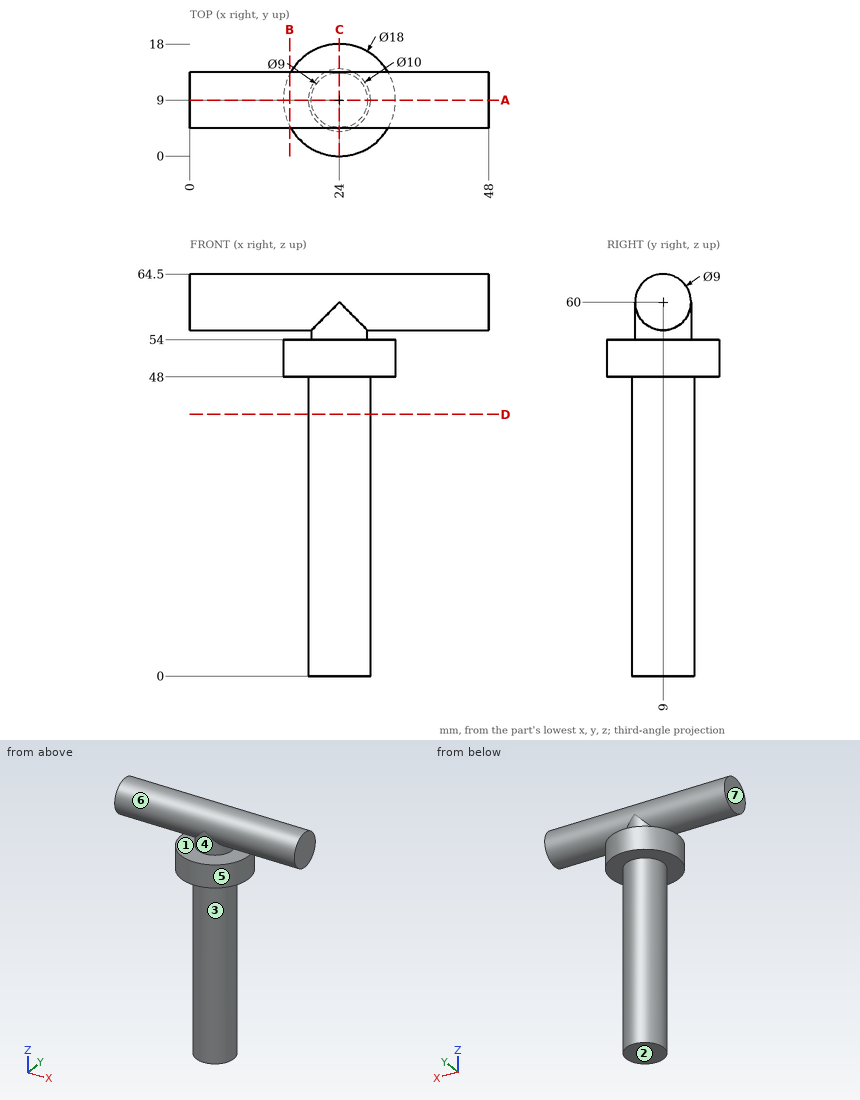
Part print with two shaded views. Sizes in mm from the minimum x, y, z corner. A direction names the side the tool comes from. Give positions to 0.01 mm unless a question says otherwise; leave off trailing zeros. Order: outer loops, then holes, each group sorted by start corner. A loop starts at its lowest first (then second) coordinate and runs counter-clockwise, first axis right, second up. Notation, with made-up numbers: M 0.5,-14.5 L 19.5,-14.5 A20 ccw 19.5,23.5 Z; hole C 16.5,38.5 d10. An arc over 180 degrees is marked long. Write item = value, one per line.
Q1. Cut at D-D, the plane z = 42. List the corners of the cut face in (x, y).
Derived:
outline = C 24,9 d10
Q2. Tool access for the marked faces 5, 6 and 7: list every direction of +Z, -Z, +X, -X, +Y, -Y with a clear straight run to the whole face (end or side of a thin tool).
Derived:
face_5 = -Z
face_6 = none
face_7 = +Z, -Z, -X, +Y, -Y
Q3. Two-plate mould, pull along Z, no slides. Class the marked faces 1, 2, 3 and 4: pulls with the +Z half, pulls with the -Z half, needs draft (parallel to the pull), parting line crosses it, or undercut.
Derived:
face_1 = undercut
face_2 = pulls with the -Z half
face_3 = needs draft
face_4 = undercut
Q4. Cut at A-A, the plane y = 9. List the corners of the cut face in (x, z), then the cut area to 3 significant figures.
Derived:
outline = M 0,55.5 L 19.5,55.5 L 19.5,54 L 15,54 L 15,48 L 19,48 L 19,0 L 29,0 L 29,48 L 33,48 L 33,54 L 28.5,54 L 28.5,55.5 L 48,55.5 L 48,64.5 L 0,64.5 Z
area = 1,030 mm2
Q5. Cut at C-C, the plane x = 24. List the corners of the cut face in (y, z), then the cut area to 3 significant figures.
Derived:
outline = M 0,48 L 4,48 L 4,0 L 14,0 L 14,48 L 18,48 L 18,54 L 13.5,54 L 13.5,60 A4.5 ccw 4.5,60 L 4.5,54 L 0,54 Z
area = 674 mm2
Q6. Cut at B-B, the plane x = 16. List the corners of the cut face in (y, z), then the cut area to 3 significant figures.
Derived:
outline = C 9,60 d9; M 4.88,48 L 13.12,48 L 13.12,54 L 4.88,54 Z
area = 113 mm2
Q7. Drill centre lines: line 1 (Z direction, x = 22.5, y = 14); line 2 (Z direction, x = 18, y = 13); line 3 (X direction, y = 8.75, z = 33.5). Where is each one in solid material? Low to high. Write a range as [from, to].
Derived:
line_1 = [48, 54]
line_2 = [48, 54], [57.94, 62.06]
line_3 = [19.01, 28.99]
Q8. Flat gauge pins, fed straight in: pin 1 (8 mm diameter, centred on x = 42.5, y = 7.5, fed in from -Z); pin 2 (6 mm diameter, centred on x = 16, y = 15.5, fed in from +Z); pin 3 (12 mm diameter, centred on x = 39.5, z = 58, fed in from -Y). Where does each tip first touch, or does it go through?
Derived:
pin_1 = 55.5
pin_2 = 62.83
pin_3 = 4.5
